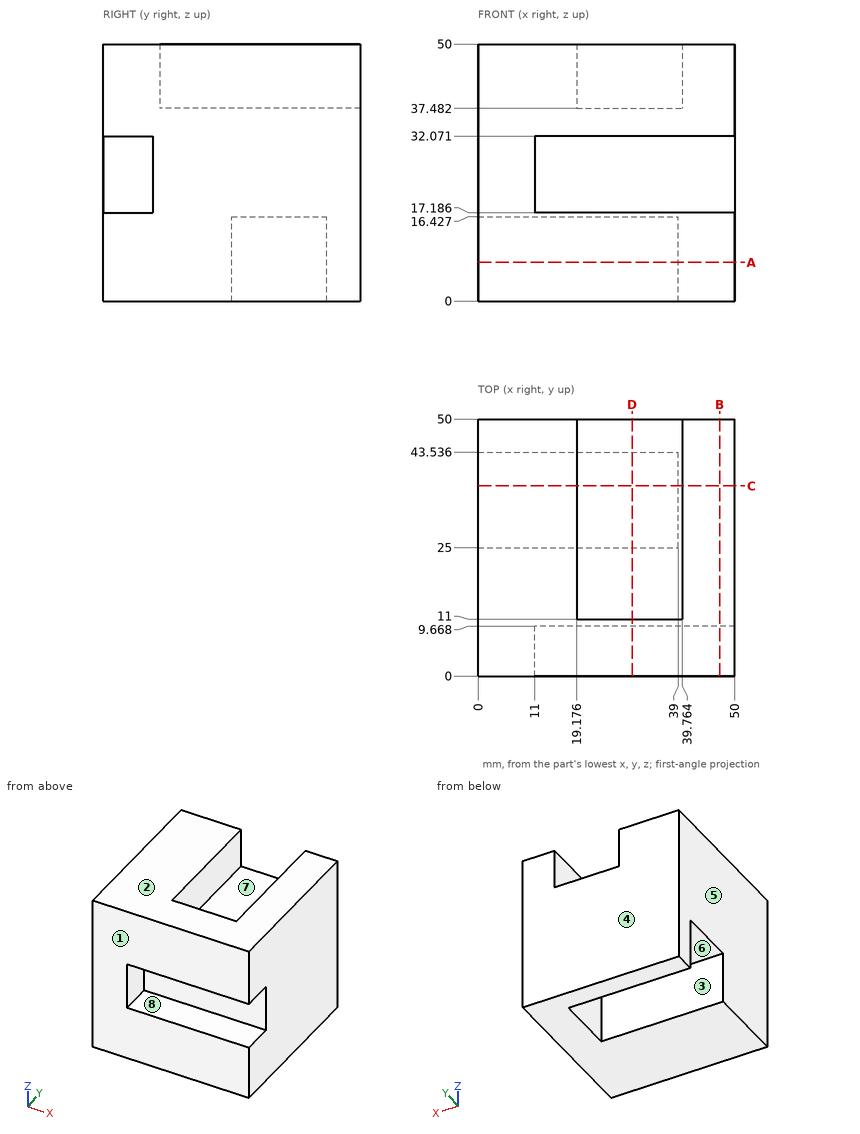
Answer from the drawing. Dimensions are ordinates in mm from the lowest x, y and z of the part. A direction names the side the tool comes from. Coordinates: 2 decimals unless noted, no trailing zeros. Loops run counter-clockwise (first coordinate to the right, second up) from the corner with the lowest first, then second, coordinate; pieces in that order, holes last. Notation, with made-up numbers: (77.5, 5.5) -> (104.5, 5.5) arc R16 cw to (104.5, 31.5) -> close; hole circle Ø7 at (43, 26). An arc over 180 degrees is marked (long way). Answer in a Markdown table with one row per item.
Item 1: For a pull along Y with two mould halves and no side action, classify the marked faces 1, 2 and 3 as released by +Y, released by -Y, zero draft, split by the parting line, or undercut.
Returned:
| item | result |
|---|---|
| face 1 | released by -Y |
| face 2 | zero draft |
| face 3 | undercut |
Item 2: A cutting plane is placed at D-D on x = 30. Determine the outline of the cut face in (y, z) (1 decimal).
Returned:
| item | result |
|---|---|
| outline | (0, 0) -> (25, 0) -> (25, 16.4) -> (43.5, 16.4) -> (43.5, 0) -> (50, 0) -> (50, 37.5) -> (11, 37.5) -> (11, 50) -> (0, 50) -> (0, 32.1) -> (9.7, 32.1) -> (9.7, 17.2) -> (0, 17.2) -> close |
Item 3: For the marked faces 4, 5, 6, 7 and 8, determine the directions among +Z, -Z, +X, -X, +Y, -Y from which every point of the face is accessible in a straight line to the end or side of a thin tool.
Returned:
| item | result |
|---|---|
| face 4 | +Z, -Z, +X, -X, +Y |
| face 5 | +Z, -Z, -X, +Y, -Y |
| face 6 | -Z, -X |
| face 7 | +Z, +Y |
| face 8 | +X, -Y |
Item 4: Each of these flat-tipped pins is pushed along its axis until it touches: P1, Ø10, axis at x = 39.5, y = 21, coming from the +Z side; P2, Ø4.5, axis at x = 35.5, z = 22, coming from the -Y side; P3, Ø6.5, axis at x = 29.5, z = 44, coming from the +Y side. Where does it stop, or does it pass through?
Returned:
| item | result |
|---|---|
| P1 | stops at z = 50 |
| P2 | stops at y = 9.67 |
| P3 | stops at y = 11 |
Item 5: A cutting plane is placed at C-C on y = 37. Determine the outline of the cut face in (x, z) (1 decimal).
Returned:
| item | result |
|---|---|
| outline | (0, 16.4) -> (39, 16.4) -> (39, 0) -> (50, 0) -> (50, 50) -> (39.8, 50) -> (39.8, 37.5) -> (19.2, 37.5) -> (19.2, 50) -> (0, 50) -> close |
Item 6: Straight lines are drawn through the part: line 1 along X through (y, z) = (14, 40.5) (1 decimal); line 2 along Y through (x, z) = (30, 10.5) (1 decimal); line 3 along Z through (x, y) = (32, 7). For each, find the intervals that lie inside material, in ascending order. Write a range as [from, to].
Returned:
| item | result |
|---|---|
| line 1 | x = [0, 19.2], [39.8, 50] |
| line 2 | y = [0, 25], [43.5, 50] |
| line 3 | z = [0, 17.19], [32.07, 50] |
Item 7: A cutting plane is placed at B-B on x = 47. Determine the outline of the cut face in (y, z), plus the area to 3 significant figures.
Returned:
| item | result |
|---|---|
| outline | (0, 0) -> (50, 0) -> (50, 50) -> (0, 50) -> (0, 32.07) -> (9.67, 32.07) -> (9.67, 17.19) -> (0, 17.19) -> close |
| area | 2,360 mm^2 |
Item 8: A cutting plane is placed at A-A on z = 7.5. Determine the outline of the cut face in (x, y) (1 decimal).
Returned:
| item | result |
|---|---|
| outline | (0, 0) -> (50, 0) -> (50, 50) -> (0, 50) -> (0, 43.5) -> (39, 43.5) -> (39, 25) -> (0, 25) -> close |
